The model under review builds one solid part; all positions refer to its coordinate system, in mm. A direction names the side the tool comes from. Round coordinates to 2 decimals unless told otherwise and drop trailing zeros. Write each loop counter-clockwise with the first axis right and the second up, starting at its lowest first coordinate (ties: lowest second). Pieces come first, ordered by that corner, then holes. Notation, with made-up numbers: M 73,6.25 L 124,6.25 A7 cw 124,10.25 Z; hole C 7,51.25 d8. An arc over 180 degrees is marked long. One line per item, written item: value. Start each with the question number.
1) Wall thickness on probe 1 along X at (y, z) = (-3, 4.5); probe 2 along Y at (x, z) = (6.5, 8.75); probe 3 along Y at (x, z) = (24, 0.75): over which ranges is each line inside the solid? List them lowest first.
2) For P1, Ø1.2, axis at y = -5.5, z = 3.5, coming from the -X side; P2, Ø2.5, axis at x = 4.5, z = 3.5, coming from the -Y side; P3, Ø4, axis at x = 29.5, z = 3, coming from the -Y side; P4, Ø3.5, axis at y = -13, z = 6.5, coming from the -X side, all flat-tipped, find the tip position at first contact; note any pin that passes through.
3) Take a section at B-B, the plane z = 4. State how many separate pieces and enclosed holes the cut face has, and give its area (3 significant figures).
4) Take a section at C-C, the plane y = -11.5. Write out the cut boundary in (x, z).
5) Take a section at A-A, the plane x = 25. Write out the cut boundary in (y, z) (3 decimals).
6) Tool access review of faces 5 (the face through (1, -6, 4)), 6 (the face through (25, 0, 1)), 7 (the face through (37, -13, 4)): name each direction out of +Z, -Z, +X, -X, +Y, -Y from which nothing blocks a thin tool from reaching the whole face with its end or side.
7) Mouldability with a two-part tool opening along X and no side actions: class faces 1 (the face through (26, -5, 0)), 2 (the face through (8, -5, 5)), 3 (the face through (44, -4.5, 5)), 4 (the face through (0, -4, 4)) as +X half, -X half, draft (parallel to the pull), parting line (faces both ways), or undercut.
from build123d import *

# Parameters (mm, degrees)
F0_R     = 9
F1_DEPTH = 9
F3_DEPTH = 50
F5_DEPTH = 3
F6_W     = 5
F6_H     = 1.5
F7_DEPTH = 25


with BuildPart() as f1:
    # F0 (on Top) → F1 (new body)
    with BuildSketch(Plane.XY):
        with BuildLine():
            Line((50, 0), (0, 0))
            Line((0, 0), (0, -6))
            Line((0, -6), (8.0002032363, -6))
            ThreePointArc((8.0002032363, -6), (11.5357371422, -7.4644660941), (13.0002032363, -11))
            Line((13.0002032363, -11), (13.0002032363, -14.9301599718))
            Line((13.0002032363, -14.9301599718), (13.0002032363, -15.0698400282))
            ThreePointArc((13.0002032363, -15.0698400282), (25.08937552, -26.9996671627), (36.9995057583, -14.8910892252))
            Line((36.9995057583, -14.8910892252), (36.9995057583, -11))
            ThreePointArc((36.9995057583, -11), (38.4639718524, -7.4644660941), (41.9995057583, -6))
            Line((41.9995057583, -6), (50, -6))
            Line((50, -6), (50, 0))
        make_face()
        with Locations((25, -15)):
            Circle(F0_R, mode=Mode.SUBTRACT)
    extrude(amount=F1_DEPTH)

    # F2 (on face) → F3 (cut)
    with BuildSketch(Plane.YZ.offset(50)):
        with BuildLine():
            Line((0, 1.375), (0, 7.625))
            ThreePointArc((0, 7.625), (-3.125, 4.5), (0, 1.375))
        make_face()
    extrude(amount=-F3_DEPTH, mode=Mode.SUBTRACT)

    # F4 (on face) → F5 (join)
    with BuildSketch(Plane.YZ.offset(50)):
        with BuildLine():
            Line((0, 1.375), (0, 0))
            ThreePointArc((0, 0), (4.5, 4.5), (0, 9))
            Line((0, 9), (0, 7.625))
            ThreePointArc((0, 7.625), (-3.125, 4.5), (0, 1.375))
        make_face()
        with BuildLine():
            ThreePointArc((0, 6.1), (1.1313708499, 5.6313708499), (1.6, 4.5))
            ThreePointArc((1.6, 4.5), (1.1313708499, 3.3686291501), (0, 2.9))
            ThreePointArc((0, 2.9), (-1.6, 4.5), (0, 6.1))
        make_face(mode=Mode.SUBTRACT)
        with BuildLine():
            Line((-6, 0), (0, 0))
            Line((0, 0), (0, 1.375))
            ThreePointArc((0, 1.375), (-3.125, 4.5), (0, 7.625))
            Line((0, 7.625), (0, 9))
            Line((0, 9), (-6, 9))
            Line((-6, 9), (-6, 0))
        make_face()
    extrude(amount=F5_DEPTH)

    # F6 (on face) → F7 (cut)
    with BuildSketch(Plane.XY.offset(9)):
        with Locations((5.5, -5.25)):
            Rectangle(F6_W, F6_H)
        with Locations((44.5, -5.25)):
            Rectangle(F6_W, F6_H)
    extrude(amount=-F7_DEPTH, mode=Mode.SUBTRACT)


solid = f1.part
Checked values:
1. probe 1: x = 50 to 53
1. probe 2: y = -4.5 to 0
1. probe 3: y = -26.96 to -23.94, -6.06 to 0
2. P1: stops at x = 0
2. P2: stops at y = -4.5
2. P3: stops at y = -26.74
2. P4: stops at x = 13
3. separate pieces: 2
3. enclosed holes: 1
3. area: 352 mm2
4. outline: M 13,0 L 16.71,0 L 16.71,9 L 13,9 Z; M 33.29,0 L 37,0 L 37,9 L 33.29,9 Z
5. outline: M -27,0 L -24,0 L -24,9 L -27,9 Z; M -6,0 L 0,0 L 0,1.375 A3.125 cw 0,7.625 L 0,9 L -6,9 Z
6. face 5: +Z, -Z, -X, -Y
6. face 6: +Z, -Z, -X, +Y
6. face 7: +Z, -Z, +X, -Y
7. face 1: draft
7. face 2: undercut
7. face 3: undercut
7. face 4: -X half
